Can you work these out from the model? Positions are in its coordinate system, mm. Face numbers are marked on the shaded views. A direction names the side the tool comes from. Give positions to 0.01 mm unless a question says otherwise; leave off trailing zeros. Loops run counter-clockwise (first coordinate to the right, second up) from the corner with the lowest first, then second, coordinate; pieces in that order, holes last. Notation, with made-up numbers: M 14,-33 L 60,-33 A15 ccw 60,-26 Z; hole C 58,10.5 d10. An arc over 180 degrees is marked long. Use CSV: the item, a comma, the result in double quotes.
from build123d import *

# Parameters (mm, degrees)
SKETCH1_R           = 1.7
BOSS_EXTRUDE1_DEPTH = 14
CUT_EXTRUDE1_DEPTH  = 4


with BuildPart() as part:
    # Sketch1 → Boss-Extrude1 (new body)
    with BuildSketch(Plane.XY):
        with BuildLine():
            Line((5.42, 5.51), (-1.71, 5.51))
            ThreePointArc((-1.71, 5.51), (-3.124213562, 4.924213562), (-3.71, 3.51))
            Line((-3.71, 3.51), (-3.71, -3.51))
            ThreePointArc((-3.71, -3.51), (-3.124213562, -4.924213562), (-1.71, -5.51))
            Line((-1.71, -5.51), (5.42, -5.51))
            ThreePointArc((5.42, -5.51), (6.834213562, -4.924213562), (7.42, -3.51))
            Line((7.42, -3.51), (7.42, 3.51))
            ThreePointArc((7.42, 3.51), (6.834213562, 4.924213562), (5.42, 5.51))
        make_face()
        Circle(SKETCH1_R, mode=Mode.SUBTRACT)
        with BuildLine():
            Line((4.21, 3.5), (4.91, 3.5))
            ThreePointArc((4.91, 3.5), (5.263553391, 3.353553391), (5.41, 3))
            Line((5.41, 3), (5.41, -3))
            ThreePointArc((5.41, -3), (5.263553391, -3.353553391), (4.91, -3.5))
            Line((4.91, -3.5), (4.21, -3.5))
            ThreePointArc((4.21, -3.5), (3.856446609, -3.353553391), (3.71, -3))
            Line((3.71, -3), (3.71, 3))
            ThreePointArc((3.71, 3), (3.856446609, 3.353553391), (4.21, 3.5))
        make_face(mode=Mode.SUBTRACT)
    extrude(amount=BOSS_EXTRUDE1_DEPTH)

    # Sketch2 → Cut-Extrude1 (cut)
    with BuildSketch(Plane.XY.offset(14)):
        Polygon((0, 3.348631561), (-2.9, 1.674315781), (-2.9, -1.674315781), (0, -3.348631561), (2.9, -1.674315781), (2.9, 1.674315781), align=None)
    extrude(amount=-CUT_EXTRUDE1_DEPTH, mode=Mode.SUBTRACT)


solid = part.part
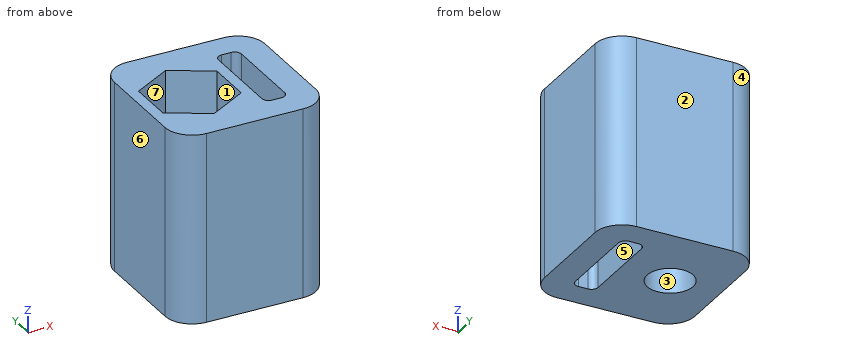
Q1. I want a section at D-D, the plane x = 0.5. Please give me the cut outline in (y, z).
Model answer:
outline,"M -5.51,0 L -1.62,0 L -1.62,10 L -3.06,10 L -3.06,14 L -5.51,14 Z; M 1.62,0 L 5.51,0 L 5.51,14 L 3.06,14 L 3.06,10 L 1.62,10 Z"
Q2. Please list where these lines run through material, in increasing order: L1, parallel to X at y = 0, z = 7; L2, parallel to X at y = -0.75, z = 13; L3, parallel to Y at x = 0, z = 2.25. Write a range as from..to.
Model answer:
L1,"-3.71..-1.7, 1.7..3.71, 5.41..7.42"
L2,"-3.71..-2.9, 2.9..3.71, 5.41..7.42"
L3,"-5.51..-1.7, 1.7..5.51"
Q3. I want a section at B-B, the plane z = 5.5. Please give me the cut outline in (x, y).
Model answer:
outline,"M -3.71,-3.51 A2 ccw -1.71,-5.51 L 5.42,-5.51 A2 ccw 7.42,-3.51 L 7.42,3.51 A2 ccw 5.42,5.51 L -1.71,5.51 A2 ccw -3.71,3.51 Z; hole C 0,0 d3.4; hole M 3.71,-3 A0.5 ccw 4.21,-3.5 L 4.91,-3.5 A0.5 ccw 5.41,-3 L 5.41,3 A0.5 ccw 4.91,3.5 L 4.21,3.5 A0.5 ccw 3.71,3 Z"
Q4. I want a section at C-C, the plane x = 4.5. Please give me the cut outline in (y, z).
Model answer:
outline,"M -5.51,0 L -3.5,0 L -3.5,14 L -5.51,14 Z; M 3.5,0 L 5.51,0 L 5.51,14 L 3.5,14 Z"
Q5. For the marked faces 5, 6 and 7, which set-ups out of +Z, -Z, +X, -X, +Y, -Y let a thin tool reach every point of the face, with its end or its side?
Model answer:
face 5,"+Z, -Z"
face 6,"+Z, -Z, -X, +Y, -Y"
face 7,"+Z"
Q6. I want a section at A-A, the plane y = 0. Please give me the cut outline in (x, z).
Model answer:
outline,"M -3.71,0 L -1.7,0 L -1.7,10 L -2.9,10 L -2.9,14 L -3.71,14 Z; M 1.7,0 L 3.71,0 L 3.71,14 L 2.9,14 L 2.9,10 L 1.7,10 Z; M 5.41,0 L 7.42,0 L 7.42,14 L 5.41,14 Z"
Q7. If we mould it in two halves opening along X, with no side actions, what happens to the marked faces 1, 2, 3 and 4? For each: released by +X, released by -X, zero draft, split by the parting line, or undercut.
Model answer:
face 1,"undercut"
face 2,"zero draft"
face 3,"undercut"
face 4,"released by -X"
Q8. I'm going to push flat-ended pins straight in: P1, Ø1.7, axis at x = 1, y = 0.5, coming from the +Z side; P2, Ø3, axis at x = 0, y = 0, coming from the -Z side. Where does each tip first touch, or does it pass through?
Model answer:
P1,"z = 10"
P2,"through"
